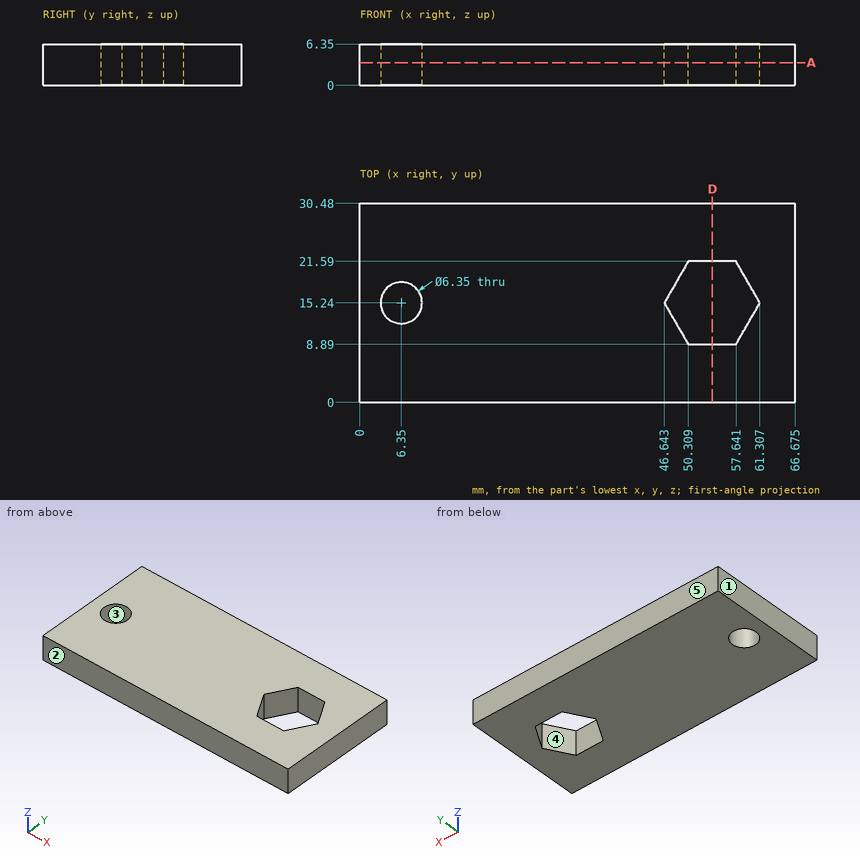
The figure shows three views and two pictorial views of one solid part (mm, origin at its lowest corner). Answer the questions. A direction names the side the tool comes from. Round coordinates to 2 decimals unless told otherwise and drop trailing zeros. Loops run counter-clockwise (first coordinate to the right, second up) from the corner with the lowest first, then second, coordinate; pieces in that order, holes last. Notation, with made-up numbers: (-22.75, 55) - (30.25, 55) arc R8 ccw to (30.25, 61) - close; hole circle Ø1 at (51, -26). An arc over 180 degrees is marked (long way). Use one line per item in the form item = value. Start each with the question number.
(1) Find section D-D on x = 54. Determine the outline of the cut face in (y, z), and give its area (3 significant figures).
(2) Determine the mould class of the marked faces 1, 2 and 3 for opening direction Y: +Y half, -Y half, draft (parallel to the pull), parting line (faces both ways), or undercut.
(3) Find section A-A on z = 3.5. Give the number of separate pieces and of enclosed holes in the cut face, and give its area (3 significant figures).
(4) Consider line 1 (Y direction, x = 56.5, z = 4.75); line 2 (Y direction, x = 6.35, z = 5.25) (1 decimal); line 3 (X direction, y = 10.5, z = 2.5) (1 decimal). Determine where each line is inside the solid, lowest interval first.
(5) Which of the six approach directions +Z, -Z, +X, -X, +Y, -Y give full straight-line access (tool end or side, diameter ignored) to the marked faces 4 and 5?
Answer list:
q1.outline = (0, 0) - (8.89, 0) - (8.89, 6.35) - (0, 6.35) - close; (21.59, 0) - (30.48, 0) - (30.48, 6.35) - (21.59, 6.35) - close
q1.area = 113 mm^2
q2.face_1 = draft
q2.face_2 = -Y half
q2.face_3 = undercut
q3.separate_pieces = 1
q3.enclosed_holes = 2
q3.area = 1,860 mm^2
q4.line_1 = 0 to 8.89, 21.59 to 30.48
q4.line_2 = 0 to 12.1, 18.4 to 30.5
q4.line_3 = 0 to 49.4, 58.6 to 66.7
q5.face_4 = +Z, -Z
q5.face_5 = +Z, -Z, +X, -X, +Y
